Work out the finished part from the listing and answer in its coordinate system (mm). Coordinates: 2 decimals unless noted, no trailing zeros. Write each loop counter-clockwise with the first axis right and the second up, starting at its lowest first coordinate (ties: lowest second). Pieces come first, ordered by that corner, then holes. Notation, with made-up numbers: (8.5, 44.5) - (39.5, 44.5) arc R13 cw to (39.5, 56.5) - close; hole circle Ø1 at (34.5, 0). An arc over 180 degrees is marked (long way). Use a Markdown table: item, result. Add a question column.
(1) For a pull along Y with two mould halves and no side action, classify faces 1 (the face through (8.1, 0, 1.5)), 2 (the face through (16.215, 26.364, 2.699)), 3 (the face through (13.09, 43.74, 0.99)) as released by +Y, released by -Y, zero draft, split by the parting line, or undercut.
(2) Find the intervals of material crossed by line 1 (Y direction, x = 3.25, z = 1.3); line 2 (X direction, y = 10, z = 2.8); line 3 (Y direction, x = 3.25, z = 0.6), in increasing order. Write a range as from..to.
(3) The part is cut by section C-C, the plane z = 2.5. Give the vertices of the cut face in (x, y), then the cut area to 3 significant figures.
(4) The part is cut by section D-D, the plane y = 17.5. Give the vertices of the cut face in (x, z), then the cut area to 3 significant figures.
(5) The part is cut by section B-B, the plane x = 3.25. Give the vertices of the cut face in (y, z), then the cut area to 3 significant figures.
(6) The part is cut by section A-A, the plane y = 9.5. State how many separate pieces and enclosed holes the cut face has, then the cut area to 3 significant figures.
(7) Given pin 1 Ø2 at (x, y) = (13.25, 9.5) entering from +Z, flat-ended and moving along its own axis, determine where the tip first touches the part or whether it passes through.
from build123d import *

# Parameters (mm, degrees)
F0_W     = 16.5
F0_H     = 52
F0_R     = 1.25
F1_DEPTH = 3
F2_R     = 0.99999


# Not quite as in the source:
# - a fillet or chamfer is up to 0.001 mm smaller than in the source, because OpenCascade refuses the exact size


with BuildPart() as f1:
    # F0 (on Top) → F1 (new body)
    with BuildSketch(Plane.XY):
        with Locations((8.25, 26)):
            Rectangle(F0_W, F0_H)
        with Locations((3.25, 9.5)):
            Circle(F0_R, mode=Mode.SUBTRACT)
        with Locations((13.25, 9.5)):
            Circle(F0_R, mode=Mode.SUBTRACT)
        with Locations((3.25, 42.5)):
            Circle(F0_R, mode=Mode.SUBTRACT)
        with Locations((13.25, 42.5)):
            Circle(F0_R, mode=Mode.SUBTRACT)
    extrude(amount=F1_DEPTH)

    # F2 (radius 1 in the source; OpenCascade refuses exactly that, so slightly less here)
    f2_edges = [f1.edges().sort_by_distance(p)[0] for p in [
        (16.5, 26, 3),
        (8.25, 52, 3),
        (0, 26, 3),
        (8.25, 0, 3),
        (2, 9.5, 3),
        (12, 9.5, 3),
        (2, 42.5, 3),
        (12, 42.5, 3),
        (16.5, 26, 0),
        (8.25, 52, 0),
        (0, 26, 0),
        (8.25, 0, 0),
    ]]
    fillet(f2_edges, radius=F2_R)


solid = f1.part
Model answer:
| question | item | result |
|---|---|---|
| 1 | face 1 | released by -Y |
| 1 | face 2 | zero draft |
| 1 | face 3 | undercut |
| 2 | line 1 | 0..8.25, 10.75..41.25, 43.75..52 |
| 2 | line 2 | 0.4..1.68, 4.82..11.68, 14.82..16.1 |
| 2 | line 3 | 0.08..8.25, 10.75..41.25, 43.75..51.92 |
| 3 | outline | (0.13, 0.13) - (16.37, 0.13) - (16.37, 51.87) - (0.13, 51.87) - close; hole circle Ø2.77 at (3.25, 9.5); hole circle Ø2.77 at (3.25, 42.5); hole circle Ø2.77 at (13.25, 9.5); hole circle Ø2.77 at (13.25, 42.5) |
| 3 | area | 816 mm^2 |
| 4 | outline | (0, 1) arc R1 ccw to (1, 0) - (15.5, 0) arc R1 ccw to (16.5, 1) - (16.5, 2) arc R1 ccw to (15.5, 3) - (1, 3) arc R1 ccw to (0, 2) - close |
| 4 | area | 48.6 mm^2 |
| 5 | outline | (0, 1) arc R1 ccw to (1, 0) - (8.25, 0) - (8.25, 2) arc R1 ccw to (7.25, 3) - (1, 3) arc R1 ccw to (0, 2) - close; (10.75, 0) - (41.25, 0) - (41.25, 2) arc R1 ccw to (40.25, 3) - (11.75, 3) arc R1 ccw to (10.75, 2) - close; (43.75, 0) - (51, 0) arc R1 ccw to (52, 1) - (52, 2) arc R1 ccw to (51, 3) - (44.75, 3) arc R1 ccw to (43.75, 2) - close |
| 5 | area | 139 mm^2 |
| 6 | separate pieces | 3 |
| 6 | enclosed holes | 0 |
| 6 | area | 32.8 mm^2 |
| 7 | pin 1 | through |
